Could you check a few things on this model? Use its own coordinates, in mm. Face numbers are marked on the shaded views. A direction names the side the tool comes from. Round coordinates to 2 decimals unless told otherwise and drop trailing zeros. Order: outer loops, then holes, each group sorted by start corner. A loop starts at its lowest first (then second) coordinate and runs counter-clockwise, first axis right, second up. Notation, with made-up numbers: (74, -9.5) - (110, -9.5) arc R15 ccw to (110, 8.5) - close; hole circle Ø7 at (48, -33.5). An arc over 180 degrees is marked (long way). Use one line per item in the form item = value.
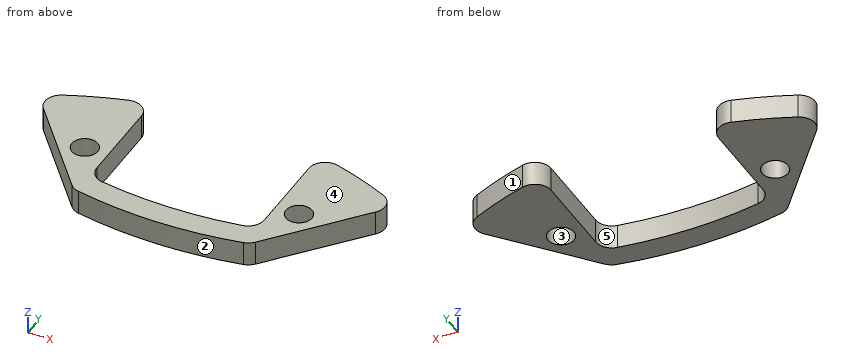
from build123d import *

# Parameters (mm, degrees)
SKETCH_1_R          = 47.75
EXTRUDE_1_DEPTH     = 3
SKETCH_2_R          = 1.6
CUT_EXTRUDE_1_DEPTH = 68.595303091
FILLET_1_R          = 2


with BuildPart() as part:
    # ｽｹｯﾁ1 → ﾎﾞｽ - 押し出し1 (new body)
    with BuildSketch(Plane.XY):
        Circle(SKETCH_1_R)
    extrude(amount=EXTRUDE_1_DEPTH)

    # ｽｹｯﾁ2 → ｶｯﾄ - 押し出し1 (cut, through all)
    with BuildSketch(Plane.XY.offset(3)):
        with Locations((-13.167775518, 36.1781659)):
            Circle(SKETCH_2_R)
        with Locations((13.167775518, 36.1781659)):
            Circle(SKETCH_2_R)
        with BuildLine():
            Line((-10.3, 46.625878008), (-10.3, 31.825692416))
            ThreePointArc((-10.3, 31.825692416), (0, 30.78), (10.3, 31.825692416))
            Line((10.3, 31.825692416), (10.3, 46.625878008))
            ThreePointArc((10.3, 46.625878008), (0, 47.75), (-10.3, 46.625878008))
        make_face()
        with BuildLine():
            Line((-22.08027891, 42.338207133), (-10.836871488, 28.938835945))
            ThreePointArc((-10.836871488, 28.938835945), (0, 27.78), (10.836871488, 28.938835945))
            Line((10.836871488, 28.938835945), (22.08027891, 42.338207133))
            ThreePointArc((22.08027891, 42.338207133), (0, -47.75), (-22.08027891, 42.338207133))
        make_face()
    extrude(amount=-CUT_EXTRUDE_1_DEPTH, mode=Mode.SUBTRACT)

    # ﾌｨﾚｯﾄ1
    fillet_1_edges = [part.edges().sort_by_distance(p)[0] for p in [
        (22.08027891, 42.338207133, 1.5),
        (-22.08027891, 42.338207133, 1.5),
        (-10.836871488, 28.938835945, 1.5),
        (10.836871488, 28.938835945, 1.5),
        (-10.3, 46.625878008, 1.5),
        (10.3, 46.625878008, 1.5),
        (10.3, 31.825692416, 1.5),
        (-10.3, 31.825692416, 1.5),
    ]]
    fillet(fillet_1_edges, radius=FILLET_1_R)


solid = part.part
Item 1: Imagine slicing it at B-B on x = 12. Please give me the cut outline in (y, z) (3 decimals), plus the area to 3 significant figures.
Found:
outline = (30.325, 0) - (35.084, 0) - (35.084, 3) - (30.325, 3) - close; (37.272, 0) - (46.043, 0) - (46.043, 3) - (37.272, 3) - close
area = 40.6 mm2
Item 2: Imagine slicing it at C-C on z = 0.8. Please give me the cut outline in (x, y), plus the area to 3 significant figures.
Found:
outline = (-20.43, 40.38) - (-11.28, 29.47) arc R2 ccw to (-10.15, 28.79) arc R51.25 ccw to (10.15, 28.79) arc R2 ccw to (11.28, 29.47) - (20.43, 40.38) arc R2 ccw to (19.73, 43.48) arc R47.75 ccw to (12.84, 45.99) arc R2 ccw to (10.3, 44.07) - (10.3, 33.48) arc R2 cw to (8.64, 31.51) arc R51.25 cw to (-8.64, 31.51) arc R2 cw to (-10.3, 33.48) - (-10.3, 44.07) arc R2 ccw to (-12.84, 45.99) arc R47.75 ccw to (-19.73, 43.48) arc R2 ccw to start; hole circle Ø3.2 at (-13.17, 36.18); hole circle Ø3.2 at (13.17, 36.18)
area = 263 mm2
Item 3: Imagine slicing it at A-A on y = 35. Please give me the cut outline in (x, z).
Found:
outline = (-15.92, 0) - (-14.25, 0) - (-14.25, 3) - (-15.92, 3) - close; (-12.09, 0) - (-10.3, 0) - (-10.3, 3) - (-12.09, 3) - close; (10.3, 0) - (12.09, 0) - (12.09, 3) - (10.3, 3) - close; (14.25, 0) - (15.92, 0) - (15.92, 3) - (14.25, 3) - close
Item 4: Imagine slicing it at D-D on y = 37.25. Please give me the cut outline in (x, z), plus the area to 3 significant figures.
Found:
outline = (-17.81, 0) - (-14.36, 0) - (-14.36, 3) - (-17.81, 3) - close; (-11.98, 0) - (-10.3, 0) - (-10.3, 3) - (-11.98, 3) - close; (10.3, 0) - (11.98, 0) - (11.98, 3) - (10.3, 3) - close; (14.36, 0) - (17.81, 0) - (17.81, 3) - (14.36, 3) - close
area = 30.8 mm2
Item 5: For the marked faces 4 and 5, which set-ups out of +Z, -Z, +X, -X, +Y, -Y let a thin tool reach every point of the face, with its end or its side?
Found:
face_4 = +Z, +X, -X, +Y, -Y
face_5 = +Z, -Z, +Y
Item 6: I need wall thicknesses on L1, parallel to X at y = 34.75, z = 2.55; L2, parallel to X at y = 39.25, z = 1.9; L3, parallel to X at y = 40, z = 1.9. Which ranges of each line are inside material? Lowest first, please.
Found:
L1 = -15.71 to -13.89, -12.45 to -10.3, 10.3 to 12.45, 13.89 to 15.71
L2 = -19.49 to -10.3, 10.3 to 19.49
L3 = -20.12 to -10.3, 10.3 to 20.12
Item 7: If we mould it in two halves opening along Y, with no side actions, what happens to the marked faces 1, 2 and 3? For each: released by +Y, released by -Y, zero draft, split by the parting line, or undercut.
Found:
face_1 = released by +Y
face_2 = released by -Y
face_3 = undercut
Item 8: Will these pins go through, and if not, where does the flat tip stop? P1, Ø0.9, axis at y = 40.5, z = 1, coming from the -X side; P2, Ø1, axis at x = -7.5, z = 0.5, coming from the -Y side.
Found:
P1 = -20.77
P2 = 28.26
